The listing builds one solid part. Answer for the finished solid, in the listing's coordinates (mm). A direction names the side the tool comes from. Coordinates: 2 decimals unless noted, no trailing zeros. Write each loop counter-clockwise with the first axis right and the second up, starting at its lowest first coordinate (ties: lowest second). Pieces come first, ordered by that corner, then holes.
```python
from build123d import *

# Parameters (mm, degrees)
SKETCH_1_R          = 2
EXTRUDE_1_DEPTH     = 3
CUT_EXTRUDE_2_DEPTH = 10
EXTRUDE_2_DEPTH     = 3
SKETCH_6_R          = 1.675
SKETCH_6_R_2        = 1.625
CUT_EXTRUDE_3_DEPTH = 85
SKETCH_7_R          = 1.675
SKETCH_7_R_2        = 1.625
CUT_EXTRUDE_4_DEPTH = 278.005212707
SKETCH_8_R          = 1.65
CUT_EXTRUDE_5_DEPTH = 10


with BuildPart() as part:
    # 草图1 → 凸台-拉伸1 (new body)
    with BuildSketch(Plane.XY):
        Polygon((-160.513239329, 50.913203436), (0, 211.426442765), (160.513239329, 50.913203436), (0, -109.600035894), align=None)
        with Locations((-32, 69.826406871)):
            Circle(SKETCH_1_R, mode=Mode.SUBTRACT)
        with Locations((32, 69.826406871)):
            Circle(SKETCH_1_R, mode=Mode.SUBTRACT)
        with Locations((0, 99.826406871)):
            Circle(SKETCH_1_R, mode=Mode.SUBTRACT)
        Polygon((-20, 0), (20, 0), (77.855339059, 57.855339059), (56.642135624, 79.068542495), (42.5, 64.926406871), (-42.5, 64.926406871), (-56.642135624, 79.068542495), (-77.855339059, 57.855339059), align=None, mode=Mode.SUBTRACT)
    extrude(amount=EXTRUDE_1_DEPTH)

    # 草图4 → 切除-拉伸2 (cut)
    with BuildSketch(Plane.XY.offset(3)):
        Polygon((-160.51323933, 65.226406871), (-160.513239329, 50.913203436), (0, -109.600035894), (160.513239329, 50.913203436), (160.513239329, 65.226406871), (-1e-09, -95.286832458), align=None)
    extrude(amount=-CUT_EXTRUDE_2_DEPTH, mode=Mode.SUBTRACT)

    # 草图5 → 凸台-拉伸2 (add)
    with BuildSketch(Plane.XY.offset(3)):
        Polygon((-1e-09, 225.739646201), (-160.51323933, 65.226406871), (-153.356637612, 58.069805153), (0, 211.426442765), (153.356637611, 58.069805154), (160.513239329, 65.226406871), align=None)
    extrude(amount=-EXTRUDE_2_DEPTH)

    # 草图6 → 切除-拉伸3 (cut)
    with BuildSketch(Plane.XY.offset(3)):
        with Locations((-1e-09, 211.597510577)):
            Circle(SKETCH_6_R)
        with Locations((73.185551852, 138.411958724)):
            Circle(SKETCH_6_R)
        with Locations((146.371103705, 65.226406871)):
            Circle(SKETCH_6_R)
        with Locations((73.185551852, -7.959144981)):
            Circle(SKETCH_6_R)
        with Locations((-1e-09, -81.144696834)):
            Circle(SKETCH_6_R)
        with Locations((-73.185551853, -7.959144981)):
            Circle(SKETCH_6_R)
        with Locations((-146.371103706, 65.226406871)):
            Circle(SKETCH_6_R)
        with Locations((-45.961940778, 165.6355698)):
            Circle(SKETCH_6_R_2)
    extrude(amount=-CUT_EXTRUDE_3_DEPTH, mode=Mode.SUBTRACT)

    # 草图7 → 切除-拉伸4 (cut, through all)
    # profile 1 of 7: a face of its own
    with BuildSketch(Plane(origin=(0, 0, 0), x_dir=(-1, 0, 0), z_dir=(0, 0, -1))):
        Polygon((-3.535533905, 186.848773236), (-21.213203435, 204.526442765), (-38.890872965, 186.848773236), (-21.213203435, 169.171103706), align=None)
    # profile 2 of 7: a face of its own
    with BuildSketch(Plane(origin=(0, 0, 0), x_dir=(-1, 0, 0), z_dir=(0, 0, -1))):
        Polygon((121.622366365, 26.335533906), (139.300035894, 44.013203436), (121.622366365, 61.690872966), (103.944696835, 44.013203436), align=None)
    # profile 3 of 7: a face of its own
    with BuildSketch(Plane(origin=(0, 0, 0), x_dir=(-1, 0, 0), z_dir=(0, 0, -1))):
        Polygon((160.51323933, 65.226406871), (80.256619665, 145.483026536), (59.04341623, 124.269823101), (121.622366365, 61.690872966), (139.300035894, 44.013203436), align=None)
        with Locations((146.371103706, 65.226406871)):
            Circle(SKETCH_7_R, mode=Mode.SUBTRACT)
    # profile 4 of 7: a face of its own
    with BuildSketch(Plane(origin=(0, 0, 0), x_dir=(-1, 0, 0), z_dir=(0, 0, -1))):
        Polygon((80.256619665, 145.483026536), (1e-09, 225.739646201), (-21.213203435, 204.526442765), (-3.535533905, 186.848773236), (59.04341623, 124.269823101), align=None)
        with Locations((45.961940778, 165.6355698)):
            Circle(SKETCH_7_R_2, mode=Mode.SUBTRACT)
        with Locations((1e-09, 211.597510577)):
            Circle(SKETCH_7_R, mode=Mode.SUBTRACT)
    # profile 5 of 7: a face of its own
    with BuildSketch(Plane(origin=(0, 0, 0), x_dir=(-1, 0, 0), z_dir=(0, 0, -1))):
        Polygon((-113.137084989, 77.247222152), (-130.814754519, 94.924891681), (-148.492424049, 77.247222152), (-130.814754519, 59.569552622), align=None)
    # profile 6 of 7: a face of its own
    with BuildSketch(Plane(origin=(0, 0, 0), x_dir=(-1, 0, 0), z_dir=(0, 0, -1))):
        Polygon((-5.656854249, -65.588347648), (-68.235804384, -3.009397513), (-130.814754519, 59.569552622), (-148.492424049, 77.247222152), (-160.513239329, 65.226406871), (1e-09, -95.286832458), (12.020815281, -83.266017178), align=None)
        with Locations((-73.185551852, -7.959144981)):
            Circle(SKETCH_7_R, mode=Mode.SUBTRACT)
        with Locations((1e-09, -81.144696834)):
            Circle(SKETCH_7_R, mode=Mode.SUBTRACT)
        with Locations((-146.371103705, 65.226406871)):
            Circle(SKETCH_7_R, mode=Mode.SUBTRACT)
    # profile 7 of 7: a face of its own
    with BuildSketch(Plane(origin=(0, 0, 0), x_dir=(-1, 0, 0), z_dir=(0, 0, -1))):
        Polygon((12.020815281, -47.910678118), (-5.656854249, -65.588347648), (12.020815281, -83.266017178), (29.69848481, -65.588347648), align=None)
    extrude(amount=-CUT_EXTRUDE_4_DEPTH, mode=Mode.SUBTRACT)

    # 草图8 → 切除-拉伸5 (cut)
    with BuildSketch(Plane(origin=(0, 0, 0), x_dir=(-1, 0, 0), z_dir=(0, 0, -1))):
        with Locations((10.606601718, 158.564501988)):
            Circle(SKETCH_8_R)
        with Locations((51.972348418, 117.198755289)):
            Circle(SKETCH_8_R)
        with Locations((93.338095117, 75.833008589)):
            Circle(SKETCH_8_R)
        with Locations((-102.530483271, 45.427416998)):
            Circle(SKETCH_8_R)
        with Locations((-61.164736572, 4.061670299)):
            Circle(SKETCH_8_R)
        with Locations((-19.798989873, -37.304076401)):
            Circle(SKETCH_8_R)
    extrude(amount=-CUT_EXTRUDE_5_DEPTH, mode=Mode.SUBTRACT)


solid = part.part
```
(1) For a pull along Y with two mould halves and no side action, classify faces 1 (the flat face through (-49.472, 71.898, 1.479)), 2 (the flat face through (85.5, 140.24, 1.52)), 3 (the flat face through (67.36, -3.886, 1.479)) as pulls with the +Y half, pulls with the -Y half, needs draft (parallel to the pull), parting line crosses it, or undercut.
(2) Section C-C, the plane x = -99 is taken. Write down the section's boundary in (y, z), plus the area to 3 significant figures.
(3) Each of these flat-tipped pins is pushed along its axis until it touches: pin 1 (1.5 mm diameter, centred on x = 11.5, z = 1, fed in from -Y); pin 2 (1.5 mm diameter, centred on x = 11, z = 1, fed in from -Y); pin 3 (0.9 mm diameter, centred on x = -3, z = 1.5, fed in from +Y). Where does it stop, or does it pass through?
(4) Which of the six approach directions +Z, -Z, +X, -X, +Y, -Y give full straight-line access (tool end or side, diameter ignored) to faces 4 (the flat face through (-3.306, -56.626, 1.479)), 5 (the flat face through (12.498, 177.886, 1.479)), 6 (the flat face through (49, 29, 1))?
(5) Section A-A, the plane x = -16.5 is taken. Write down the section's boundary in (y, z).
(6) Find the intervals of material crossed by probe 1 along Y at (x, z) = (0, 2.25); probe 2 along X at (y, z) = (73.5, 0.2); probe 3 along Y at (x, z) = (20.5, 1), in increasing order.
(7) Section B-B, the plane z = 1.25 is taken. State how many separate pieces and enclosed holes the cut face has, plus the area to 3 significant figures.
Solution:
1. face 1: undercut
1. face 2: pulls with the +Y half
1. face 3: pulls with the -Y half
2. outline: (3.71, 0) - (84.31, 0) - (84.31, 3) - (3.71, 3) - close
2. area: 242 mm2
3. pin 1: stops at y = -60.5
3. pin 2: stops at y = -61
3. pin 3: stops at y = 180.76
4. face 4: +Z, -Z, -Y
4. face 5: +Z, -Z, +Y
4. face 6: +Z, -Z
5. outline: (-52.39, 0) - (0, 0) - (0, 3) - (-52.39, 3) - close; (64.93, 0) - (166.81, 0) - (166.81, 3) - (64.93, 3) - close
6. probe 1: y = -59.93 to 0, 64.93 to 97.83, 101.83 to 183.31
6. probe 2: x = -109.81 to -62.21, -51.07 to 51.07, 62.21 to 116.88
6. probe 3: y = -50.75 to -38.8, -35.81 to 0.5, 64.93 to 169.88
7. separate pieces: 1
7. enclosed holes: 12
7. area: 31,100 mm2
